Autodesk Inventor part; units mm, degrees
ref_plane "YZ Plane" through (0, 0, 0) normal (1, 0, 0) x (0, 1, 0)
ref_plane "XZ Plane" through (0, 0, 0) normal (0, 1, 0) x (-1, 0, 0)
ref_plane "XY Plane" through (0, 0, 0) normal (0, 0, 1) x (1, 0, 0)
sketch "Sketch1" plane through (0, 0, 0) normal (0, 0, 1) x (1, 0, 0)
  line L0 (-8.1504, 12.0476) -> (-8.1504, 5.6976)
  line L1 (-8.1504, 5.6976) -> (-14.5004, 5.6976)
  line L2 (-14.5004, 5.6976) -> (-14.5004, -7.0024)
  line L3 (-14.5004, -7.0024) -> (-3.0704, -7.0024)
  line L4 (-3.0704, -7.0024) -> (-3.0704, -13.3524)
  line L5 (-3.0704, -13.3524) -> (-1.8004, -13.3524)
  line L6 (-1.8004, 12.0476) -> (-8.1504, 12.0476)
  line L7 (-1.8004, 12.0476) -> (-1.8004, -13.3524)
  dimension "d0" = 12.7
  dimension "d1" = 6.35
  dimension "d3" = 1.27
  dimension "d8" = 12.7
  dimension "d9" = 6.35
revolve "Revolution1" add sketch "Sketch1" angle 360 about axis through (-1.8004, 12.0476, 0) along (0, -1, 0)
properties part number "roll2"
Geometry check sheet. Reference: the model listing, model coordinates, mm. A direction names the side the tool comes from. Give positions to 0.01 mm unless a question says otherwise; leave off trailing zeros. Write each loop counter-clockwise with the first axis right and the second up, starting at its lowest first coordinate (ties: lowest second). Pieces come first, ordered by that corner, then holes. Notation, with made-up numbers: M 80.25,19 L 104.25,19 A10 cw 104.25,30 Z; hole C 42.25,55 d7. An arc over 180 degrees is marked long. Answer as CSV lines item,"result". Start each with the question number.
Q1. Section check B-B, the plane x = 0.25. Record the cut outline in (y, z).
Q2. Section check D-D, the plane z = -9.25. Record the cut outline in (x, y), then the cut area to 3 significant figures.
Q3. Go/stop test with flat-tipped pins: pin 1 (12 mm diameter, centred on x = 1, y = -0.5, fed in from +Z); pin 2 (1.5 mm diameter, centred on y = -0.5, z = -5, fed in from +X); pin 3 (1 mm diameter, centred on x = -5, y = -4.5, fed in from +Z); pin 4 (5 mm diameter, centred on y = 5.5, z = 3, fed in from -X). Record where each tip stops, or that it passes through.
Q4. Section check C-C, the plane y = 5. Record the cut outline in (x, z), then the cut area to 3 significant figures.
Q5. Material ranges on L1, parallel to Y at x = -12.25, z = -0.5; L2, parallel to Y at x = 1.5, z = 1; L3, parallel to X at y = 9, z = -0.25, recorded low to high.
Q6. Tool access check on faces 1 (the face through (4, 5.698, 3)), 2 (the face through (-1.64, -10.22, -1.26)), 3 (the face through (-2, -13.352, 0)). Record the directions out of +Z, -Z, +X, -X, +Y, -Y that give a thin tool (end or side, any length) a straight path to the whole face; none if there is none.
Q7. Section check A-A, the plane z = 0. Record the cut outline in (x, y).
Geometry says:
1,outline,"M -7,-12.53 L 5.7,-12.53 L 5.7,-6.01 L 12.05,-6.01 L 12.05,6.01 L 5.7,6.01 L 5.7,12.53 L -7,12.53 Z"
2,outline,"M -10.5,-7 L 6.9,-7 L 6.9,5.7 L -10.5,5.7 Z"
2,area,"221 mm^2"
3,pin 1,"z = 12.7"
3,pin 2,"x = 10.17"
3,pin 3,"z = 12.41"
3,pin 4,"x = -14.49"
4,outline,"C -1.8,0 d25.4"
4,area,"507 mm^2"
5,L1,"-7 to 5.7"
5,L2,"-7 to 12.05"
5,L3,"-8.15 to 4.54"
6,face 1,"+Y"
6,face 2,"-Y"
6,face 3,"+Z, -Z, +X, -X, -Y"
7,outline,"M -14.5,-7 L -3.07,-7 L -3.07,-13.35 L -0.53,-13.35 L -0.53,-7 L 10.9,-7 L 10.9,5.7 L 4.55,5.7 L 4.55,12.05 L -8.15,12.05 L -8.15,5.7 L -14.5,5.7 Z"
